Part model, mm, in its own coordinate system. Round coordinates to 2 decimals unless told otherwise and drop trailing zeros. Write each loop counter-clockwise with the first axis right and the second up, starting at its lowest first coordinate (ties: lowest second). Pieces come first, ordered by that corner, then holes.
```python
from build123d import *

# Parameters (mm, degrees)
SKETCH1_R      = 1.5
EXTRUDE1_DEPTH = 2.5


with BuildPart() as part:
    # Sketch1 → Extrude1 (new body)
    with BuildSketch(Plane(origin=(0, 0, 0), x_dir=(1, 0, 0), z_dir=(0, 1, 0))):
        Polygon((-3.175426481, 0), (-1.58771324, 2.75), (1.58771324, 2.75), (3.175426481, 0), (1.58771324, -2.75), (-1.58771324, -2.75), align=None)
        with Locations(Location((0, 0, 0), (0, 0, 270))):  # turned: the seam where the file's is
            Circle(SKETCH1_R, mode=Mode.SUBTRACT)
    extrude(amount=EXTRUDE1_DEPTH)

    # Sketch2 → Cut-Revolve1 (revolve, cut)
    with BuildSketch(Plane.XY, mode=Mode.PRIVATE) as cut_revolve1_sk:
        Polygon((1.5, 2.5), (1.8, 2.5), (1.5, 2.2), align=None)
        Polygon((1.5, 0), (1.8, 0), (1.5, 0.3), align=None)
        Polygon((3.175426481, 0), (3.175426481, 0.18097998), (2.5, 0), align=None)
        Polygon((3.175426481, 2.5), (3.175426481, 2.31902002), (2.5, 2.5), align=None)
    revolve(cut_revolve1_sk.sketch.rotate(Axis((0, 0, 0), (0, 1, 0)), 90), axis=Axis((0, 0, 0), (0, 1, 0)), mode=Mode.SUBTRACT)  # turned: the seam where the file's is


solid = part.part
```
Q1. Cut at A-A on x = 0. Write the cut outline in (y, z).
Values follow:
outline: (0, -2.5) - (0.07, -2.75) - (2.43, -2.75) - (2.5, -2.5) - (2.5, -1.8) - (2.2, -1.5) - (0.3, -1.5) - (0, -1.8) - close; (0, 1.8) - (0.3, 1.5) - (2.2, 1.5) - (2.5, 1.8) - (2.5, 2.5) - (2.43, 2.75) - (0.07, 2.75) - (0, 2.5) - close
Q2. Wall check: L1, parallel to Z at x = 0.25, y = 0.55; L2, parallel to Z at x = 1, y = 0.6; L3, parallel to X at y = 1.4, z = -1.3. Give the ranges that are in metal, low to high.
Values follow:
L1: z = -2.75 to -1.48, 1.48 to 2.75
L2: z = -2.75 to -1.12, 1.12 to 2.75
L3: x = -2.42 to -0.75, 0.75 to 2.42
Q3. Mould opens along X. For faces 1 (the cylindrical face through (0.45, 1.24, 1.43)), 2 (the flat face through (-2.39, 1.23, -1.36)), 3 (the flat face through (2.39, 1.23, 1.36)) say: +X half, -X half, draft (parallel to the pull), parting line (faces both ways), or undercut.
Values follow:
face 1: undercut
face 2: -X half
face 3: +X half
Q4. Drop a flat-ended pin along its axis: pin 1 (1.5 mm diameter, centred on y = 0.5, z = -1, fed in from -X). Give the stop position or say it passes through.
Values follow:
pin 1: stops at x = -3.03
Q5. Cut at B-B on y = 0.55. Write the cut outline in (x, z), plus the area to 3 significant figures.
Values follow:
outline: (-3.18, 0) - (-1.59, -2.75) - (1.59, -2.75) - (3.18, 0) - (1.59, 2.75) - (-1.59, 2.75) - close; hole circle Ø3 at (0, 0)
area: 19.1 mm2
